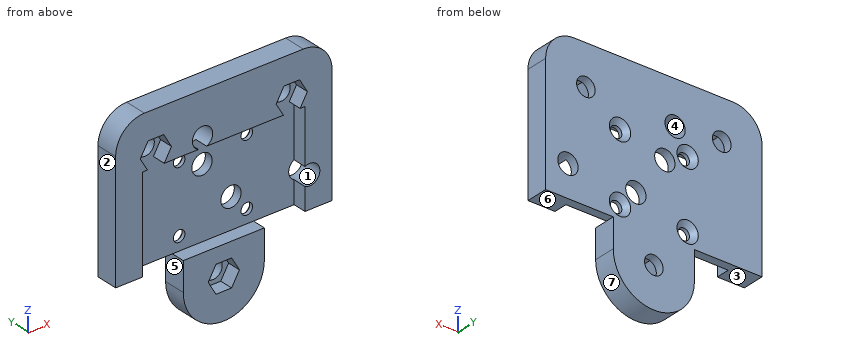
Autodesk Fusion 360 part; units mm, degrees
sketch "Sketch1" plane through (0, 0, 0) normal (0, 1, 0) x (1, 0, 0)
  circle A0 centre (0, 0) radius 12
  line L0 (32, -52) -> (-32, -52)
  line L1 (-32, -52) -> (-32, -8.5)
  line L2 (-32, -8.5) -> (32, -8.5)
  line L3 (32, -8.5) -> (32, -52)
  line L4 (0, 0) -> (0, -52) construction
  line L5 (-12, 0) -> (-12, -8.5)
  line L6 (12, 0) -> (12, -8.5)
  dimension "d1" = 24
  dimension "d2" = 64
  dimension "d3" = 43.5
  dimension "d4" = 64
extrude "Extrude1" add sketch "Sketch1" along normal blind 6.5
fillet "Fillet1" radius 8.5 2 edges at (-32, 3.25, 52) (32, 3.25, 52)
sketch "Sketch2" plane through (0, 0, 0) normal (0, -1, 0) x (1, 0, 0)
  line L0 (-12, 8.5) -> (-12, 0)
  arc A0 (-12, 0) -> (12, 0) centre (0, 0) ccw
  line L1 (12, 0) -> (12, 8.5)
  line L2 (12, 8.5) -> (32, 8.5)
  line L3 (32, 8.5) -> (32, 43.5)
  line L4 (23.5, 52) -> (-23.5, 52)
  line L5 (-32, 43.5) -> (-32, 8.5)
  line L6 (-32, 8.5) -> (-12, 8.5)
  line L7 (-32, 40.215) -> (32, 40.215) construction
  circle A1 centre (-20.1, 40.215) radius 2.5 construction
  circle A2 centre (0, 0) radius 2.5 construction
  circle A3 centre (20.1, 40.215) radius 2.5 construction
  line L8 (0, 0) -> (0, 48) construction
  line L9 (-17.7906, 36.215) -> (-15.4812, 40.215)
  line L10 (-15.4812, 40.215) -> (-17.7906, 44.215)
  line L11 (-17.7906, 44.215) -> (-22.4094, 44.215)
  line L12 (-22.4094, 44.215) -> (-24.7188, 40.215)
  line L13 (-24.7188, 40.215) -> (-22.4094, 36.215)
  line L14 (-22.4094, 36.215) -> (-17.7906, 36.215)
  line L15 (22.4094, 36.215) -> (24.7188, 40.215)
  line L16 (24.7188, 40.215) -> (22.4094, 44.215)
  line L17 (22.4094, 44.215) -> (17.7906, 44.215)
  line L18 (17.7906, 44.215) -> (15.4812, 40.215)
  line L19 (15.4812, 40.215) -> (17.7906, 36.215)
  line L20 (17.7906, 36.215) -> (22.4094, 36.215)
  line L21 (2.3094, -4) -> (4.6188, 0)
  line L22 (4.6188, 0) -> (2.3094, 4)
  line L23 (2.3094, 4) -> (-2.3094, 4)
  line L24 (-2.3094, 4) -> (-4.6188, 0)
  line L25 (-4.6188, 0) -> (-2.3094, -4)
  line L26 (-2.3094, -4) -> (2.3094, -4)
  arc A4 (32, 43.5) -> (23.5, 52) centre (23.5, 43.5) ccw
  arc A5 (-23.5, 52) -> (-32, 43.5) centre (-23.5, 43.5) ccw
  point P0 (-20.1, 40.215)
  point P1 (20.1, 40.215)
  dimension "d7" = 40.215
  dimension "d8" = 5
  dimension "d9" = 5
  dimension "d10" = 5
  dimension "d11" = 20.1
  dimension "d12" = 20.1
  dimension "d13" = 4
  dimension "d14" = 4
  dimension "d45" = 4
hole "Hole1" at (-20.1, 0, 40.215) at (20.1, 0, 40.215) at (0, 0, 0) direction (0, 1, 0) diameter 5.5 depth 16 tip angle 118
sketch "Sketch3" plane through (0, 0, 0) normal (0, -1, 0) x (1, 0, 0)
  circle A0 centre (20.1, 40.215) radius 2.75
  circle A1 centre (-20.1, 40.215) radius 2.75
  circle A2 centre (0, 0) radius 2.75
  line L0 (-12, 8.5) -> (-12, 0)
  arc A3 (-12, 0) -> (12, 0) centre (0, 0) ccw
  line L1 (12, 0) -> (12, 8.5)
  line L2 (12, 8.5) -> (32, 8.5)
  line L3 (32, 8.5) -> (32, 43.5)
  line L4 (23.5, 52) -> (-23.5, 52)
  line L5 (-32, 43.5) -> (-32, 8.5)
  line L6 (-32, 8.5) -> (-12, 8.5)
  line L7 (0, 0) -> (0, 52) construction
  line L8 (32, 0) -> (-32, 0) construction
  circle A4 centre (5.32, 17.45) radius 3
  circle A5 centre (25.4, 17.815) radius 3
  circle A6 centre (-3.25, 29.2) radius 3
  circle A7 centre (-6.3, 39.25) radius 3
  arc A8 (32, 43.5) -> (23.5, 52) centre (23.5, 43.5) ccw
  arc A9 (-23.5, 52) -> (-32, 43.5) centre (-23.5, 43.5) ccw
  dimension "d18" = 6
  dimension "d19" = 17.45
  dimension "d20" = 5.32
  dimension "d21" = 6
  dimension "d22" = 25.4
  dimension "d23" = 17.815
  dimension "d24" = 6
  dimension "d25" = 6
  dimension "d26" = 6.3
  dimension "d27" = 3.25
  dimension "d28" = 39.25
  dimension "d29" = 29.2
extrude "Extrude2" cut sketch "Sketch3" against normal through all contours A4 | A5 | A6 | A7
sketch "Sketch4" plane through (0, 0, 0) normal (0, -1, 0) x (1, 0, 0)
  circle A0 centre (5.32, 17.45) radius 3
  circle A1 centre (-3.25, 29.2) radius 3
  circle A2 centre (25.4, 17.815) radius 3
  circle A3 centre (-6.3, 39.25) radius 3
  circle A4 centre (20.1, 40.215) radius 2.75
  circle A5 centre (-20.1, 40.215) radius 2.75
  circle A6 centre (0, 0) radius 2.75
  line L0 (-12, 8.5) -> (-12, 0)
  arc A7 (-12, 0) -> (12, 0) centre (0, 0) ccw
  line L1 (12, 0) -> (12, 8.5)
  line L2 (12, 8.5) -> (32, 8.5)
  line L3 (32, 8.5) -> (32, 43.5)
  line L4 (23.5, 52) -> (-23.5, 52)
  line L5 (-32, 43.5) -> (-32, 8.5)
  line L6 (-32, 8.5) -> (-12, 8.5)
  line L7 (0, 56) -> (0, 0) construction
  line L8 (41, 0) -> (0, 0) construction
  line L9 (24, 8.5) -> (-24, 8.5)
  line L10 (-24, 8.5) -> (-24, 36.5)
  line L11 (-24, 36.5) -> (24, 36.5)
  line L12 (24, 36.5) -> (24, 8.5)
  line L13 (24, 8.5) -> (-24, 36.5) construction
  line L14 (-24, 8.5) -> (24, 36.5) construction
  line L15 (10, 32.5) -> (-10, 32.5) construction
  line L16 (-10, 32.5) -> (-10, 12.5) construction
  line L17 (-10, 12.5) -> (10, 12.5) construction
  line L18 (10, 12.5) -> (10, 32.5) construction
  line L19 (10, 32.5) -> (-10, 12.5) construction
  line L20 (-10, 32.5) -> (10, 12.5) construction
  arc A8 (32, 43.5) -> (23.5, 52) centre (23.5, 43.5) ccw
  arc A9 (-23.5, 52) -> (-32, 43.5) centre (-23.5, 43.5) ccw
  point P0 (0, 22.5)
  point P1 (0, 22.5)
  dimension "d31" = 48
  dimension "d32" = 28
  dimension "d33" = 20
  dimension "d34" = 20
  dimension "d35" = 8.5
extrude "Extrude3" cut sketch "Sketch4" against normal blind 4 contours A2 A3 L2 L6 L9 L10 L11 L12 | A3 L11 picked at (-6.5707, 36.454)
extrude "Extrude4" cut sketch "Sketch2" against normal blind 4 contours L9 L10 L11 L12 L13 L14 | L15 L16 L17 L18 L19 L20 | L21 L22 L23 L24 L25 L26
sketch "Sketch5" plane through (0, 6.5, 0) normal (0, 1, 0) x (-1, 0, 0)
  circle A0 centre (-5.32, 17.45) radius 3
  circle A1 centre (3.25, 29.2) radius 3
  circle A2 centre (-25.4, 17.815) radius 3
  circle A3 centre (6.3, 39.25) radius 3
  circle A4 centre (-20.1, 40.215) radius 2.75
  circle A5 centre (20.1, 40.215) radius 2.75
  circle A6 centre (0, 0) radius 2.75
  line L0 (12, 0) -> (12, 8.5)
  line L1 (12, 8.5) -> (32, 8.5)
  line L2 (32, 8.5) -> (32, 43.5)
  line L3 (23.5, 52) -> (-23.5, 52)
  line L4 (-32, 43.5) -> (-32, 8.5)
  line L5 (-32, 8.5) -> (-12, 8.5)
  line L6 (-12, 8.5) -> (-12, 0)
  arc A7 (-12, 0) -> (12, 0) centre (0, 0) ccw
  line L7 (-10, 32.5) -> (10, 32.5)
  line L8 (-10, 12.5) -> (-10, 32.5)
  line L9 (10, 32.5) -> (10, 12.5)
  line L10 (10, 12.5) -> (-10, 12.5)
  arc A8 (-23.5, 52) -> (-32, 43.5) centre (-23.5, 43.5) ccw
  arc A9 (32, 43.5) -> (23.5, 52) centre (23.5, 43.5) ccw
hole "Hole2" at (10, 6.5, 32.5) at (10, 6.5, 12.5) at (-10, 6.5, 12.5) at (-10, 6.5, 32.5) direction (0, -1, 0) diameter 3.4 depth 16 tip angle 118 countersink diameter 6.3 countersink angle 90
CAD build for the part. Positions are in the model's coordinates, mm. Face numbers are marked on the shaded views. A direction names the side the tool comes from. Round coordinates to 2 decimals unless told otherwise and drop trailing zeros. Order: outer loops, then holes, each group sorted by start corner. A loop starts at its lowest first (then second) coordinate and runs counter-clockwise, first axis right, second up. Notation, with made-up numbers: M 84.25,66.25 L 112.25,66.25 A23 cw 112.25,78.25 Z; hole C 65,72.5 d3. An arc over 180 degrees is marked long. Use one line per item in the form item = value.
Q1. Two-plate mould, pull along Z, no slides. Class the marked faces 1, 2, 3 and 4: +Z half, -Z half, draft (parallel to the pull), parting line (faces both ways), or undercut.
Recorded:
face_1 = undercut
face_2 = draft
face_3 = -Z half
face_4 = undercut
Q2. Saw through at B-B on x = 20.1. Give the cut face in (y, z) (3 decimals), then the cut area to 3 significant figures.
Recorded:
outline = M 0,44.215 L 4,44.215 L 4,42.965 L 6.5,42.965 L 6.5,52 L 0,52 Z; M 4,8.5 L 6.5,8.5 L 6.5,37.465 L 4,37.465 Z
area = 126 mm^2
Q3. Saw through at D-D on y = 1.5. State how many separate pieces and enclosed holes the cut face has, then the cut area to 3 significant figures.
Recorded:
separate_pieces = 2
enclosed_holes = 1
area = 1,630 mm^2
Q4. Saw through at C-C on x = -1. Give the cut face in (y, z).
Recorded:
outline = M 0,-11.96 L 6.5,-11.96 L 6.5,-2.56 L 4,-2.56 L 4,-4 L 0,-4 Z; M 0,4 L 4,4 L 4,2.56 L 6.5,2.56 L 6.5,27.22 L 4,27.22 L 4,8.5 L 0,8.5 Z; M 0,36.5 L 4,36.5 L 4,31.18 L 6.5,31.18 L 6.5,52 L 0,52 Z
Q5. Saw through at A-A on z = 12.5. Give the cut face in (x, y), then the cut area to 3 significant figures.
Recorded:
outline = M -32,0 L -24,0 L -24,4 L -11.7,4 L -11.7,5.05 L -13.15,6.5 L -32,6.5 Z; M -8.3,4 L 8.3,4 L 8.3,5.05 L 6.85,6.5 L -6.85,6.5 L -8.3,5.05 Z; M 11.7,4 L 24,4 L 24,0 L 32,0 L 32,6.5 L 13.15,6.5 L 11.7,5.05 Z
area = 203 mm^2
Q6. Which spindle directions (+Z, -Z, +X, -X, +Y, -Y) get a long thin tool onto all of the face, cutting with end or side? Do the marked faces 5, 6 and 7. Say none if no direction does.
Recorded:
face_5 = -Z, -X, +Y, -Y
face_6 = -Z, +X, +Y, -Y
face_7 = -Z, +Y, -Y
Q7. Probe L1, parallel to X at y = 2, z = 24; L2, parallel to Z at x = 0, y = 5.5; L3, parallel to Z at x = 20.1, y = 5.4 (3 decimals). List the from-to ranges inside material, lowest first.
Recorded:
L1 = -32 to -24, 24 to 32
L2 = -12 to -2.75, 2.75 to 52
L3 = 8.5 to 37.465, 42.965 to 52
Q8. Flat gauge pins, fed straight in: P1, Ø2.5, axis at x = -10, z = 12.5, coming from the -Y side; P2, Ø6.5, axis at x = 20.1, z = 40.215, coming from the -Y side; P3, Ø1.5, axis at x = 25.5, y = 3.5, coming from the +Z side; P4, Ø0.7, axis at x = -23, y = 2.5, coming from the -Z side. Where does each tip first touch, or does it go through?
Recorded:
P1 = through
P2 = 4
P3 = 51.91
P4 = 36.5
